Input: dimensioned drawing with shaded views. Units: mm. Origin: part minimum x, y, z. A direction names the side the tool comes from. Round coordinates to 2 decimals unless told otherwise and drop trailing zeros. Order: outer loops, then holes, each group sorted by start corner. A loop starts at its lowest first (then second) coordinate and runs counter-clockwise, first axis right, second up.
Item 1: Line query: L1, parallel to Y at x = 5, z = 6; L2, parallel to Z at x = 2.25, y = 8; L3, parallel to X at y = 6.75, z = 7.75. Output: solid intervals per line, ascending.
Item 2: First-contact query: pin 1 (4 mm diameter, centred on x = 6.5, y = 6.5, fed in from -Z); pin 2 (1.5 mm diameter, centred on y = 2.5, z = 8, fed in from -X); pin 3 (3 mm diameter, centred on y = 6.5, z = 5.5, fed in from -X); pin 4 (1 mm diameter, centred on y = 8.5, z = 2.5, fed in from +X). Flat tips, straight axial feed; report the tip coordinate or a pass-through.
Item 3: Cut plane D-D on z = 8.5. Output: boundary loops of the cut face in (x, y), then the cut area to 3 significant figures.
Item 4: Reachability of the marked faces 1 and 2 from +Z, -Z, +X, -X, +Y, -Y: full face, straight path, thin tool, end or side. Return the list, or none.
Item 5: Cut plane A-A on y = 5. Output: boundary loops of the cut face in (x, z).
Item 6: Cut plane C-C on z = 2. Output: boundary loops of the cut face in (x, y).
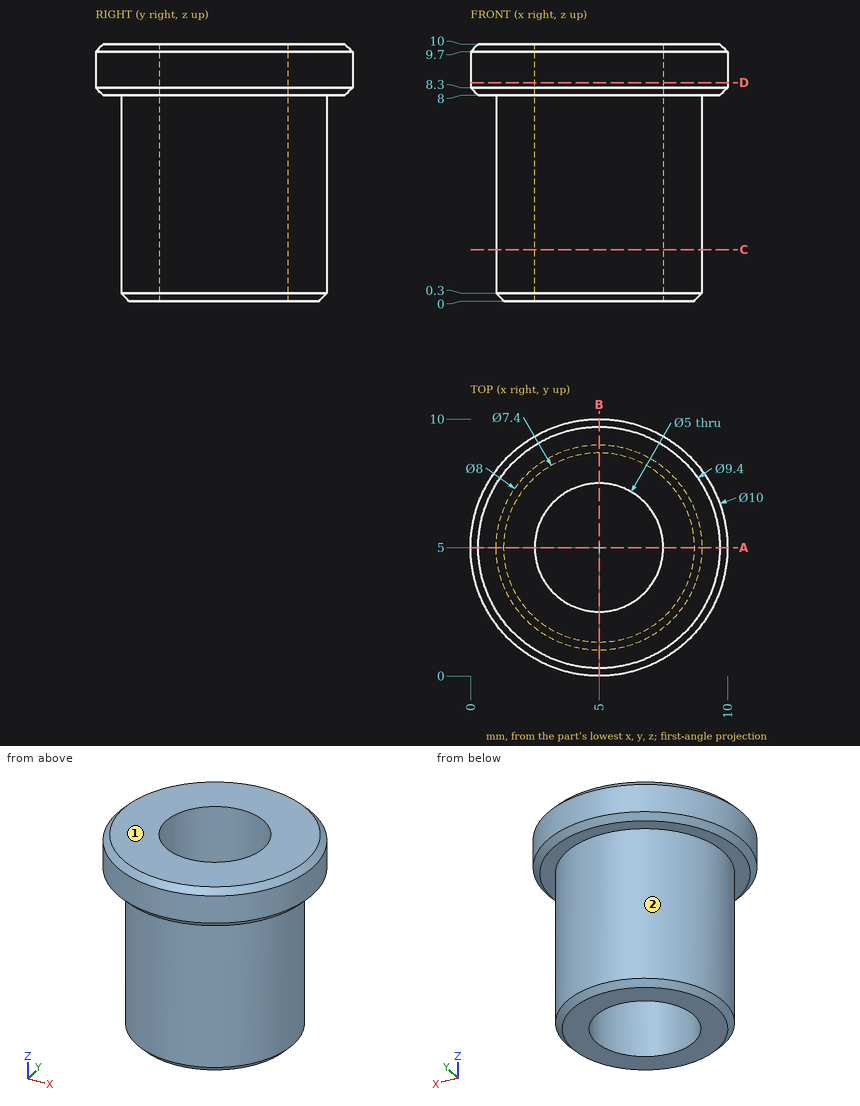
From the geometry:
1. L1: y = 1 to 2.5, 7.5 to 9
1. L2: z = 8 to 10
1. L3: x = 1.4 to 3.21, 6.79 to 8.6
2. pin 1: stops at z = 0
2. pin 2: stops at x = 0.34
2. pin 3: stops at x = 1
2. pin 4: stops at x = 7.65
3. outline: circle Ø10 at (5, 5); hole circle Ø5 at (5, 5)
3. area: 58.9 mm2
4. face 1: +Z, +X, -X, +Y, -Y
4. face 2: -Z
5. outline: (0, 8.3) - (0.3, 8) - (1, 8) - (1, 0.3) - (1.3, 0) - (2.5, 0) - (2.5, 10) - (0.3, 10) - (0, 9.7) - close; (7.5, 0) - (8.7, 0) - (9, 0.3) - (9, 8) - (9.7, 8) - (10, 8.3) - (10, 9.7) - (9.7, 10) - (7.5, 10) - close
6. outline: circle Ø8 at (5, 5); hole circle Ø5 at (5, 5)
